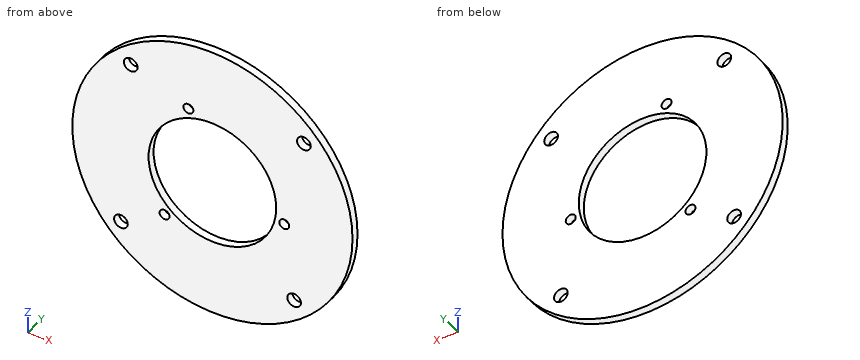
```python
from build123d import *

# Parameters (mm, degrees)
F0_R     = 57.15
F1_DEPTH = 3.175
F2_R     = 2.794
F3_DEPTH = 25.4
F4_R     = 26.035
F4_R_2   = 2.032
F5_DEPTH = 25.4


with BuildPart() as f1:
    # F0 (on Front) → F1 (new body)
    with BuildSketch(Plane.XZ):
        Circle(F0_R)
    extrude(amount=F1_DEPTH)

    # F2 (on face) → F3 (cut)
    with BuildSketch(Plane.XZ.offset(3.175)):
        with Locations((-33.326707, 37.324684)):
            Circle(F2_R)
        with Locations((-37.324684, -33.326707)):
            Circle(F2_R)
        with Locations((33.326707, -37.324684)):
            Circle(F2_R)
        with Locations((37.324684, 33.326707)):
            Circle(F2_R)
    extrude(amount=-F3_DEPTH, mode=Mode.SUBTRACT)

    # F4 (on face) → F5 (cut)
    with BuildSketch(Plane.XZ.offset(3.175)):
        Circle(F4_R)
        with Locations((-9.790665, 28.193384)):
            Circle(F4_R_2)
        with Locations((-19.520854, -22.575657)):
            Circle(F4_R_2)
        with Locations((29.311519, -5.617728)):
            Circle(F4_R_2)
    extrude(amount=-F5_DEPTH, mode=Mode.SUBTRACT)


solid = f1.part
```
Source: CAD feature listing. Evaluate the final solid. Frame: model axes, mm. Give positions to 0.01 mm unless a question says otherwise; leave off trailing zeros. Write each loop counter-clockwise with the first axis right and the second up, starting at its lowest first coordinate (ties: lowest second). Pieces come first, ordered by that corner, then holes. Notation, with made-up numbers: (43.5, 53.25) - (91.5, 53.25) arc R32 ccw to (91.5, 80.25) - close; hole circle Ø9 at (52.5, 19.5). An arc over 180 degrees is marked (long way). One line per item, written item: value. Start each with the question number.
Q1. First-contact query: pin 1 Ø1 at (x, y) = (12, -1.5) entering from -Z. Flat tip, straight axial feed; report the tip coordinate or a pass-through.
Q2. Section query D-D, the plane z = -47. Return the cut outline in (x, y) (3 decimals).
Q3. Material intervals for probe 1 along X at (y, z) = (-1.4, -21); probe 2 along X at (y, z) = (-0.45, 4.5); probe 3 along X at (y, z) = (-1.5, -11), sorted ascending. Write a range as from..to.
Q4. Section query A-A, the plane z = 0. Return the cut outline in (x, y) (3 decimals).
Q5. Section query C-C, the plane y = -1.35. Count the separate pieces of the cut face and the enclosed holes in it, then the cut area to 3 significant figures.
Q6. Section query B-B, the plane x = 0. Return the cut outline in (y, z) (3 decimals).
Answer:
1. pin 1: stops at z = -55.98
2. outline: (-32.513, -3.175) - (32.513, -3.175) - (32.513, 0) - (-32.513, 0) - close
3. probe 1: x = -53.15..-20.8, -18.24..-15.39, 15.39..53.15
3. probe 2: x = -56.97..-25.64, 25.64..56.97
3. probe 3: x = -56.08..-23.6, 23.6..56.08
4. outline: (-57.15, -3.175) - (-26.035, -3.175) - (-26.035, 0) - (-57.15, 0) - close; (26.035, -3.175) - (57.15, -3.175) - (57.15, 0) - (26.035, 0) - close
5. separate pieces: 1
5. enclosed holes: 8
5. area: 7,990 mm2
6. outline: (-3.175, -57.15) - (0, -57.15) - (0, -26.035) - (-3.175, -26.035) - close; (-3.175, 26.035) - (0, 26.035) - (0, 57.15) - (-3.175, 57.15) - close
